Geometry: final body of the model. Coordinates: model frame, mm. A direction names the side the tool comes from. Give positions to 0.01 mm unless a question says otherwise; leave off trailing zeros. Write each loop counter-clockwise with the first axis right and the second up, starting at its lowest first coordinate (ties: lowest second). Pieces come first, ordered by that corner, then holes. Notation, with made-up numbers: M -34.75,-38 L -8.75,-38 A20 cw -8.75,-8 Z; hole C -10.5,75.25 d8. An arc over 180 degrees is marked long. Use a Markdown table: item, result. Add a question column.
1) Draft query along Z for faces 3 (the flat face through (2, 15, 5)), 4 (the cylindrical face through (1.73, 6.11, -7.81)), 5 (the flat face through (0, 0, 0)). Return one class per face: +Z half, -Z half, draft (parallel to the pull), parting line (faces both ways), or undercut.
2) Section A-A on y = 1.75. Return the cut outline in (x, z), then the cut area to 3 significant figures.
3) Line query: line 1 (X direction, y = 6.5, z = 0.25); line 2 (Z direction, x = 0, y = 5.25); line 3 (Z direction, x = 4.25, y = 5). Output: solid intervals per line, ascending.
4) Section B-B on z = 0. Return the cut outline in (x, y).
5) Set-up query: faces 1 (the flat face through (0, -3, 0)), 2 (the cylindrical face through (1.08, 7.4, 4.88)). Return all of +Z, -Z, +X, -X, +Y, -Y with unobstructed straight access to the full face (end or side cutting, diameter ignored); none if empty.
6) Pin query (flat end, axial travel): pin 1 (2 mm diameter, centred on y = 5.5, z = 5, fed in from +X); pin 2 (2 mm diameter, centred on y = 3, z = -5, fed in from -X); pin 3 (3 mm diameter, centred on x = -3, y = 5.5, fed in from +Z). Return the tip coordinate at first contact, or that it passes through.
7) Section C-C on x = 0. Return the cut outline in (y, z).
8) Section D-D on y = -1.5. Return the cut outline in (x, z).
Autodesk Inventor part; units mm, degrees
ref_plane "YZ Plane" through (0, 0, 0) normal (1, 0, 0) x (0, 1, 0)
ref_plane "XZ Plane" through (0, 0, 0) normal (0, 1, 0) x (-1, 0, 0)
ref_plane "XY Plane" through (0, 0, 0) normal (0, 0, 1) x (1, 0, 0)
sketch "Sketch1" plane through (0, 0, 0) normal (0, 1, 0) x (-1, 0, 0)
  circle A0 centre (0, 0) radius 5
  circle A1 centre (0, 0) radius 8
  dimension "d0" = 10
  dimension "d1" = 16
extrude "Extrusion1" add sketch "Sketch1" against normal blind 3 contours A0 | A1
extrude "Extrusion2" add sketch "Sketch1" along normal blind 15
chamfer "Chamfer1" distance 1 angle 45 2 edges at (8, 15, 0) (8, -3, 0)
properties part number "3DP_ASA_Rod_End_Cap"
Found:
| question | item | result |
|---|---|---|
| 1 | face 3 | draft |
| 1 | face 4 | parting line |
| 1 | face 5 | undercut |
| 2 | outline | C 0,0 d16; hole C 0,0 d10 |
| 2 | area | 123 mm² |
| 3 | line 1 | -8 to -4.99, 4.99 to 8 |
| 3 | line 2 | -8 to -5, 5 to 8 |
| 3 | line 3 | -6.78 to -2.63, 2.63 to 6.78 |
| 4 | outline | M -8,-2 L -7,-3 L 7,-3 L 8,-2 L 8,14 L 7,15 L 5,15 L 5,0 L -5,0 L -5,15 L -7,15 L -8,14 Z |
| 5 | face 1 | +Z, -Z, +X, -X, -Y |
| 5 | face 2 | +Y |
| 6 | pin 1 | x = 6.93 |
| 6 | pin 2 | x = -6.93 |
| 6 | pin 3 | z = 7.86 |
| 7 | outline | M -3,-7 L -2,-8 L 14,-8 L 15,-7 L 15,-5 L 0,-5 L 0,5 L 15,5 L 15,7 L 14,8 L -2,8 L -3,7 Z |
| 8 | outline | C 0,0 d16 |
